Input: part model. Units: mm. Frame: model coordinates. A direction names the side the tool comes from. Coordinates: 2 decimals unless noted, no trailing zeros.
from build123d import *

# Parameters (mm, degrees)
F0_W     = 600
F0_H     = 400
F1_DEPTH = 220
F2_R     = 20
F4_DEPTH = 15
F7_DEPTH = 26
F8_W     = 570
F8_H     = 370
F9_DEPTH = 114
F9_TAPER = 2


with BuildPart() as f1:
    # F0 (on Top) → F1 (new body)
    with BuildSketch(Plane.XY):
        with Locations((8.6124254986, 0)):
            Rectangle(F0_W, F0_H)
    extrude(amount=F1_DEPTH)

    # F2
    f2_edges = [f1.edges().sort_by_distance(p)[0] for p in [
        (-291.387575, -200, 110),
        (308.612425, -200, 110),
        (308.612425, 200, 110),
        (-291.387575, 200, 110),
    ]]
    fillet(f2_edges, radius=F2_R)

    # F3 (on face) → F4 (cut)
    with BuildSketch(Plane(origin=(0, 0, 0), x_dir=(1, 0, 0), z_dir=(0, 0, -1))):
        with BuildLine():
            ThreePointArc((308.6124254986, 180), (302.7545611224, 194.1421356237), (288.6124254986, 200))
            Line((288.6124254986, 200), (-271.3875745014, 200))
            ThreePointArc((-271.3875745014, 200), (-285.5297101251, 194.1421356237), (-291.3875745014, 180))
            Line((-291.3875745014, 180), (-291.3875745014, -180))
            ThreePointArc((-291.3875745014, -180), (-285.5297101251, -194.1421356237), (-271.3875745014, -200))
            Line((-271.3875745014, -200), (288.6124254986, -200))
            ThreePointArc((288.6124254986, -200), (302.7545611224, -194.1421356237), (308.6124254986, -180))
            Line((308.6124254986, -180), (308.6124254986, 180))
        make_face()
        with BuildLine():
            ThreePointArc((-275.0983515568, 177.5), (-273.6338854627, 181.0355339059), (-270.0983515568, 182.5))
            Line((-270.0983515568, 182.5), (284.9016484432, 182.5))
            ThreePointArc((284.9016484432, 182.5), (288.4371823491, 181.0355339059), (289.9016484432, 177.5))
            Line((289.9016484432, 177.5), (289.9016484432, -177.5))
            ThreePointArc((289.9016484432, -177.5), (288.4371823491, -181.0355339059), (284.9016484432, -182.5))
            Line((284.9016484432, -182.5), (-270.0983515568, -182.5))
            ThreePointArc((-270.0983515568, -182.5), (-273.6338854627, -181.0355339059), (-275.0983515568, -177.5))
            Line((-275.0983515568, -177.5), (-275.0983515568, 177.5))
        make_face(mode=Mode.SUBTRACT)
    extrude(amount=-F4_DEPTH, mode=Mode.SUBTRACT)

    # F6 (on offset) → F7 (cut)
    with BuildSketch(Plane.XY.offset(216.5)):
        with BuildLine():
            ThreePointArc((-271.3875745014, 200), (-285.5297101251, 194.1421356237), (-291.3875745014, 180))
            Line((-291.3875745014, 180), (-291.3875745014, -180))
            ThreePointArc((-291.3875745014, -180), (-285.5297101251, -194.1421356237), (-271.3875745014, -200))
            Line((-271.3875745014, -200), (288.6124254986, -200))
            ThreePointArc((288.6124254986, -200), (302.7545611224, -194.1421356237), (308.6124254986, -180))
            Line((308.6124254986, -180), (308.6124254986, 180))
            ThreePointArc((308.6124254986, 180), (302.7545611224, 194.1421356237), (288.6124254986, 200))
            Line((288.6124254986, 200), (-271.3875745014, 200))
        make_face()
        with BuildLine():
            ThreePointArc((-278.3875745014, 180), (-276.3373219697, 184.9497474683), (-271.3875745014, 187))
            Line((-271.3875745014, 187), (288.6124254986, 187))
            ThreePointArc((288.6124254986, 187), (293.5621729669, 184.9497474683), (295.6124254986, 180))
            Line((295.6124254986, 180), (295.6124254986, -180))
            ThreePointArc((295.6124254986, -180), (293.5621729669, -184.9497474683), (288.6124254986, -187))
            Line((288.6124254986, -187), (-271.3875745014, -187))
            ThreePointArc((-271.3875745014, -187), (-276.3373219697, -184.9497474683), (-278.3875745014, -180))
            Line((-278.3875745014, -180), (-278.3875745014, 180))
        make_face(mode=Mode.SUBTRACT)
    extrude(amount=-F7_DEPTH, mode=Mode.SUBTRACT)

    # F8 (on face) → F9 (cut)
    with BuildSketch(Plane.XY.offset(220)):
        with Locations((8.6124254986, 0)):
            Rectangle(F8_W, F8_H)
    extrude(amount=-F9_DEPTH, taper=F9_TAPER, mode=Mode.SUBTRACT)


solid = f1.part
Item 1: Draft query along Z for faces 1 (the face through (7, -6, 106)), 2 (the face through (-285.68, -193.99, 103.98)), 3 (the face through (5, 187, 204)). Return one class per face: pulls with the +Z half, pulls with the -Z half, needs draft (parallel to the pull), parting line crosses it, or undercut.
Response values:
face 1: pulls with the +Z half
face 2: needs draft
face 3: undercut
Item 2: Ray query, probe 1 along Y at (x, z) = (-230, 147.5); probe 2 along Z at (x, y) = (142, -101.5); probe 3 along X at (y, z) = (144, 174). Return the intervals inside material, ascending.
Response values:
probe 1: y = -200 to -182.47, 182.47 to 200
probe 2: z = 0 to 106
probe 3: x = -291.39 to -274.78, 292.01 to 308.61
Item 3: Pin query (flat end, axial travel): pin 1 Ø16.5 at (y, z) = (46.5, 10.5) entering from +X; pin 2 Ø5 at (x, y) = (103, 50.5) entering from +Z; pin 3 Ø4.5 at (x, z) = (44, 6.5) entering from -Y; pin 4 Ø16.5 at (x, z) = (38.5, 5) entering from +Y. Return the tip coordinate at first contact, or that it passes through.
Response values:
pin 1: stops at x = 308.61
pin 2: stops at z = 106
pin 3: stops at y = -182.5
pin 4: stops at y = 182.5
Item 4: Access query for faces 4 (the face through (289.902, -2, 7)), 5 (the face through (4, -182.5, 7)), 6 (the face through (-278.388, -3, 204)). Directions: +Z, -Z, +X, -X, +Y, -Y. A direction counts if a zero-diameter tool reaches every point of the face in a straight line with its end or side. Return the directions, or none.
Response values:
face 4: -Z, +X, +Y, -Y
face 5: -Z, +X, -X, -Y
face 6: -X, +Y, -Y
